Geometry: final body of the model. Coordinates: model frame, mm. Face numbers are marked on the shaded views. A direction names the side the tool comes from. Coordinates: 2 decimals unless noted, no trailing zeros. Write each loop counter-clockwise with the first axis right and the second up, starting at its lowest first coordinate (ties: lowest second). Pieces come first, ordered by that corner, then holes. Notation, with made-up numbers: M 17,25 L 44,25 A16 ccw 44,44 Z; hole C 57,-26.5 d9. An arc over 180 degrees is marked long. Write item = value, one per line. Start each with the question number.
Item 1: Section C-C on z = -34. Output: boundary loops of the cut face in (x, y), plus the area to 3 significant figures.
Item 2: Section A-A on z = -7. Output: boundary loops of the cut face in (x, y).
Item 3: Section B-B on x = 0. Give the number of separate pieces and of enclosed holes in the cut face, plus the area to 3 significant figures.
Item 4: Ray query, L1, parallel to Z at x = -16, y = -17; L2, parallel to Y at x = -1, z = -8.5; L3, parallel to X at y = -12, z = -2. Return the intervals inside material, ascending. Write a range as [from, to].
Item 5: Reachability of the marked faces 4 and 5 from +Z, -Z, +X, -X, +Y, -Y: full face, straight path, thin tool, end or side. Return the list, or none.
Item 6: First-contact query: pin 1 Ø1.5 at (x, y) = (-22, 12.7) entering from +Z; pin 2 Ø12 at (x, z) = (10, -29.5) entering from +Y; pin 3 Ø3 at (y, z) = (12, -13.5) entering from -X. Flat tips, straight axial feed; report the tip coordinate or a pass-through.
Item 7: Pull-direction query (Y, two-part tool) for the marked faces 1, 2 and 3; classes: +Y half, -Y half, draft (parallel to the pull), parting line (faces both ways), or undercut.
from build123d import *

# Parameters (mm, degrees)
M3X0_5_TAPPED_HOLE1_D     = 2.5
M3X0_5_TAPPED_HOLE1_DEPTH = 10
SKETCH5_R                 = 22.73
SKETCH5_R_2               = 20.5
CUT_EXTRUDE1_DEPTH        = 1.32


with BuildPart() as part:
    # Sketch1 → Revolve1 (revolve)
    with BuildSketch(Plane(origin=(0, 0, 0), x_dir=(1, 0, 0), z_dir=(0, 1, 0))):
        Polygon((-28.58, 0), (-28.58, 10), (-25.06, 10), (-25.06, 16), (-23.03, 16), (-23.03, 19.56), (-25.06, 19.56), (-25.06, 24.56), (-23.03, 24.56), (-23.03, 28.12), (-25.06, 28.12), (-25.06, 33.12), (-23.03, 33.12), (-23.03, 36.68), (-25.06, 36.68), (-25.06, 41.68), (-17.03, 41.68), (-17.03, 0), align=None)
    revolve(axis=Axis((0, 0, 0), (0, 0, -1)))

    # M3x0.5 Tapped Hole1
    with Locations(Plane.XY):
        with Locations((0, 25.4), (21.997045256, 12.7), (21.997045256, -12.7), (0, -25.4), (-21.997045256, -12.7), (-21.997045256, 12.7)):
            Hole(M3X0_5_TAPPED_HOLE1_D / 2, depth=M3X0_5_TAPPED_HOLE1_DEPTH)

    # Sketch5 → Cut-Extrude1 (cut)
    with BuildSketch(Plane.XY):
        Circle(SKETCH5_R)
        Circle(SKETCH5_R_2, mode=Mode.SUBTRACT)
    extrude(amount=-CUT_EXTRUDE1_DEPTH, mode=Mode.SUBTRACT)


solid = part.part
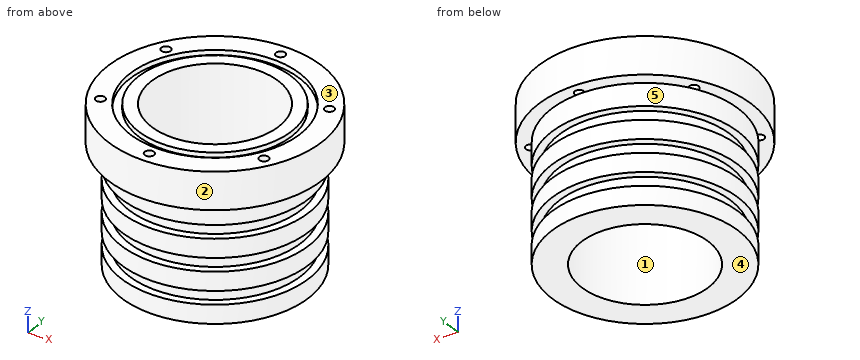
Responses:
q1.outline = C 0,0 d46.06; hole C 0,0 d34.06
q1.area = 755 mm²
q2.outline = C 0,0 d57.16; hole C -22,-12.7 d2.5; hole C -22,12.7 d2.5; hole C 0,0 d34.06; hole C 0,-25.4 d2.5; hole C 0,25.4 d2.5; hole C 22,-12.7 d2.5; hole C 22,12.7 d2.5
q3.separate_pieces = 4
q3.enclosed_holes = 0
q3.area = 641 mm²
q4.L1 = [-41.68, -36.68], [-33.12, -28.12], [-24.56, -19.56], [-16, 0]
q4.L2 = [-28.56, -26.15], [-24.65, -17], [17, 24.65], [26.15, 28.56]
q4.L3 = [-25.94, -23.03], [-20.96, -12.08], [12.08, 20.96], [23.03, 25.94]
q5.face_4 = -Z, +X, -X, +Y, -Y
q5.face_5 = -Z
q6.pin_1 = -10
q6.pin_2 = 24.74
q6.pin_3 = -22.75
q7.face_1 = undercut
q7.face_2 = parting line
q7.face_3 = draft
